Could you check a few things on this model? Use its own coordinates, in mm. Face numbers are marked on the shaded views. A direction names the side the tool comes from. Give positions to 0.01 mm unless a question says otherwise; leave off trailing zeros. Loops run counter-clockwise (first coordinate to the right, second up) from the corner with the lowest first, then second, coordinate; pieces in that order, holes last. Notation, with made-up numbers: (-28.75, 64) -> (24.25, 64) arc R31 cw to (24.25, 102) -> close; hole circle Ø8 at (51, 47). An arc over 180 degrees is marked (long way). Put each result on its own line as item: value.
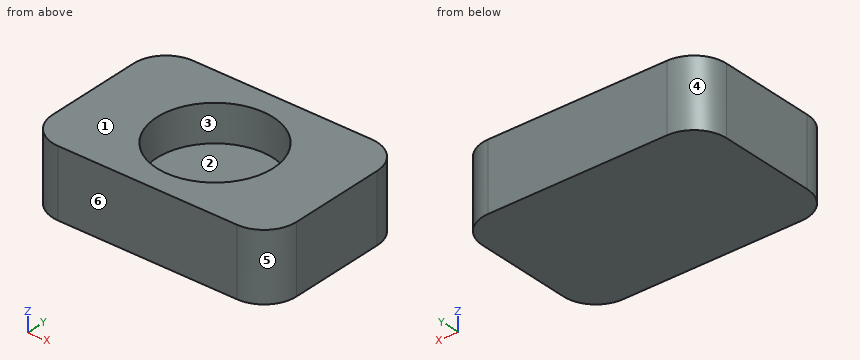
```python
from build123d import *

# Parameters (mm, degrees)
F0_W     = 30
F0_H     = 19.9
F1_DEPTH = 8.3
F2_R     = 7.15
F3_DEPTH = 4.52
F4_R     = 4


with BuildPart() as f1:
    # F0 (on Top) → F1 (new body)
    with BuildSketch(Plane.XY):
        with Locations((-1.016058, -4.658131)):
            Rectangle(F0_W, F0_H)
    extrude(amount=F1_DEPTH)

    # F2 (on face) → F3 (cut)
    with BuildSketch(Plane.XY.offset(8.3)):
        with Locations((-1.016058, -4.658131)):
            Circle(F2_R)
    extrude(amount=-F3_DEPTH, mode=Mode.SUBTRACT)

    # F4
    f4_edges = [f1.edges().sort_by_distance(p)[0] for p in [
        (13.983942, -14.608131, 4.15),
        (-16.016058, -14.608131, 4.15),
        (13.983942, 5.291869, 4.15),
        (-16.016058, 5.291869, 4.15),
    ]]
    fillet(f4_edges, radius=F4_R)


solid = f1.part
```
1. I need wall thicknesses on line 1 (X direction, y = -10, z = 5.25); line 2 (X direction, y = -7.75, z = 5.5); line 3 (Y direction, x = 3.5, z = 7). Which ranges of each line are inside material? Lowest first, please.
Recorded:
line 1: x = -16.02 to -5.77, 3.74 to 13.98
line 2: x = -16.02 to -7.46, 5.43 to 13.98
line 3: y = -14.61 to -10.2, 0.89 to 5.29
2. For the marked faces 1 and 2, which set-ups out of +Z, -Z, +X, -X, +Y, -Y let a thin tool reach every point of the face, with its end or its side?
Recorded:
face 1: +Z, +X, -X, +Y, -Y
face 2: +Z
3. If we section it at C-C (y = -0.5): List the corners of the cut face in (x, z) for me, then the cut area to 3 significant figures.
Recorded:
outline: (-16.02, 0) -> (13.98, 0) -> (13.98, 8.3) -> (4.8, 8.3) -> (4.8, 3.78) -> (-6.83, 3.78) -> (-6.83, 8.3) -> (-16.02, 8.3) -> close
area: 196 mm^2
4. Thinking about a two-plate mould opening in X: for the marked faces 3, 4, 5 and 6, which applies, pulls with the +X half, pulls with the -X half, needs draft (parallel to the pull), parting line crosses it, or undercut?
Recorded:
face 3: undercut
face 4: pulls with the -X half
face 5: pulls with the +X half
face 6: needs draft
5. If we section it at B-B (x = -5.5): List the corners of the cut face in (y, z) for me.
Recorded:
outline: (-14.61, 0) -> (5.29, 0) -> (5.29, 8.3) -> (0.91, 8.3) -> (0.91, 3.78) -> (-10.23, 3.78) -> (-10.23, 8.3) -> (-14.61, 8.3) -> close
6. If we section it at D-D (x = -14): List the corners of the cut face in (y, z) for me.
Recorded:
outline: (-14.08, 0) -> (4.77, 0) -> (4.77, 8.3) -> (-14.08, 8.3) -> close
7. If we section it at A-A (z = 6): List the corners of the cut face in (x, y) for me, then the cut area to 3 significant figures.
Recorded:
outline: (-16.02, -10.61) arc R4 ccw to (-12.02, -14.61) -> (9.98, -14.61) arc R4 ccw to (13.98, -10.61) -> (13.98, 1.29) arc R4 ccw to (9.98, 5.29) -> (-12.02, 5.29) arc R4 ccw to (-16.02, 1.29) -> close; hole circle Ø14.3 at (-1.02, -4.66)
area: 423 mm^2
